from build123d import *

# Parameters (mm, degrees)
CHAMFER_1_SIZE = 1
CHAMFER_2_SIZE = 0.1
CHAMFER_3_SIZE = 0.3


with BuildPart() as part:
    # 스케치1 → 회전1 (revolve)
    with BuildSketch(Plane(origin=(0, 0, 0), x_dir=(0, 0, -1), z_dir=(1, 0, 0))):
        with BuildLine():
            Line((4.2, 0), (4.2, 1))
            Line((4.2, 1), (4.2, 7))
            Line((4.2, 7), (4.7, 7.500000078))
            Line((4.7, 7.500000078), (4.7, 8.000000078))
            Line((4.7, 8.000000078), (4.2, 8.5))
            Line((4.2, 8.5), (4.2, 10))
            Line((4.2, 10), (4.7, 10.500000078))
            Line((4.7, 10.500000078), (4.7, 11.000000078))
            Line((4.7, 11.000000078), (4.2, 11.5))
            Line((4.2, 11.5), (4.2, 13))
            Line((4.2, 13), (4.7, 13.500000078))
            Line((4.7, 13.500000078), (4.7, 14.000000078))
            Line((4.7, 14.000000078), (4.2, 14.5))
            Line((4.2, 14.5), (4.2, 28))
            Line((4.2, 28), (3.533728258, 29.430530536))
            Line((3.533728258, 29.430530536), (2.802745502, 31))
            Line((2.802745502, 31), (2.399244734, 31.778552392))
            ThreePointArc((2.399244734, 31.778552392), (2.719290067, 32.253174869), (2.946609162, 32.778552392))
            Line((2.946609162, 32.778552392), (3.229990685, 33.260397004))
            Line((3.229990685, 33.260397004), (3.229990685, 33.62037773))
            Line((3.229990685, 33.62037773), (3.02, 33.830368416))
            Line((3.02, 33.830368416), (3.02, 34.830368416))
            Line((3.02, 34.830368416), (3.189631584, 35))
            Line((3.189631584, 35), (6, 35))
            Line((6, 35), (6, 25))
            Line((6, 25), (11.05, 10))
            Line((11.05, 10), (11.05, 8))
            Line((11.05, 8), (10.05, 8))
            Line((10.05, 8), (9.5, 7))
            Line((9.5, 7), (9.5, 5))
            Line((9.5, 5), (10.075, 5))
            Line((10.075, 5), (10.075, 1))
            Line((10.075, 1), (9.5, -0.374573668))
            Line((9.5, -0.374573668), (9.5, -2))
            Line((9.5, -2), (4.2, -2))
            Line((4.2, -2), (4.2, 0))
        make_face()
    revolve(axis=Axis((0, 0, 0), (0, 1, 0)))

    # 모따기1
    chamfer_1_edges = [part.edges().sort_by_distance(p)[0] for p in [
        (0, 35, 6),
        (0, -2, 4.2),
    ]]
    chamfer(chamfer_1_edges, length=CHAMFER_1_SIZE)

    # 모따기2
    # the kernel refuses this chamfer: 0.191354542, 0.1 mm, written as the material it takes off along each edge
    with BuildSketch(Plane(origin=(0, 31.778552392, 0), x_dir=(0, 0, -1), z_dir=(1, 0, 0))) as chamfer_2_piece_1:
        with BuildLine():
            Line((2.52619809, 0.166311611), (2.399244734 + CHAMFER_2_SIZE * 0.460143640426, -CHAMFER_2_SIZE * 0.887844485355))
            Line((2.399244734 + CHAMFER_2_SIZE * 0.460143640426, -CHAMFER_2_SIZE * 0.887844485355), (2.399244734, 0))
            ThreePointArc((2.399244734, 0), (2.466310937, 0.08495162), (2.52619809, 0.166311611))
        make_face()
    revolve(axis=Axis((0, 31.778552392, 0), (0, 1, 0)), mode=Mode.SUBTRACT)

    # 모따기3
    chamfer_3_edges = [part.edges().sort_by_distance(p)[0] for p in [
        (0, 8, 11.05),
    ]]
    chamfer(chamfer_3_edges, length=CHAMFER_3_SIZE)


solid = part.part
For this review, take the finished solid that the model builds, in its own axes (mm). A direction names the side the tool comes from. Coordinates: 2 decimals unless noted, no trailing zeros. Loops run counter-clockwise (first coordinate to the right, second up) from the corner with the lowest first, then second, coordinate; pieces in that order, holes last. Notation, with made-up numbers: (-24, 24) - (-10, 24) arc R33 ccw to (-10, 62) - close; hole circle Ø5 at (12, 62). An arc over 180 degrees is marked (long way). Return JSON: item names as keys, results as strings.
Item 1: Mouldability with a two-part tool opening along Z and no side actions: class faces 4 (the cylindrical face through (1.237, 33.443, -2.984)), 5 (the cylindrical face through (-1.262, 9.26, -4.006)), 6 (the cylindrical face through (0, 29, 6)), 7 (the flat face through (1, 35, 3.3)) as pulls with the +Z half, pulls with the -Z half, needs draft (parallel to the pull), parting line crosses it, or undercut.
Determined:
{"face 4": "undercut", "face 5": "undercut", "face 6": "parting line crosses it", "face 7": "needs draft"}
Item 2: Take a section at B-B (y = 16). Give the boundary of the cut face in (x, z), then the cut area to 3 significant figures.
Determined:
{"outline": "circle Ø18.06 at (0, 0); hole circle Ø8.4 at (0, 0)", "area": "201 mm2"}
Item 3: For line 1 (Z direction, x = 0, y = 9); line 2 (X direction, y = 7.6, z = 0); line 3 (Z direction, x = -2.75, y = 1), list the stretches that pass through material, from the lowest coordinate up.
Determined:
{"line 1": "z = -11.05 to -4.2, 4.2 to 11.05", "line 2": "x = -9.83 to -4.7, 4.7 to 9.83", "line 3": "z = -9.69 to -3.17, 3.17 to 9.69"}
Item 4: Insertion check: pin 1 (10 mm diameter, centred on y = 23, z = 5.5, fed in from +X); pin 2 (9.5 mm diameter, centred on x = 0, z = 0, fed in from -Y); pin 3 (7 mm diameter, centred on x = 0, z = 0, fed in from -Y). Each pin has a flat end and moves straight along its axis. Give the tip position at first contact, or say it passes through.
Determined:
{"pin 1": "stops at x = 7.63", "pin 2": "stops at y = -1.55", "pin 3": "stops at y = 29.5"}
Item 5: For faces 1 (the flat face through (9, 5, 4)), 2 (the cylindrical face through (8.43, -1.2, -4.38)), 3 (the flat face through (4, -2, -4)), list the 3-axis set-ups (+Z, -Z, +X, -X, +Y, -Y) from which the entire face can be reached by the end or side of a thin tool; tool diameter is ignored.
Determined:
{"face 1": "none", "face 2": "-Y", "face 3": "+Z, -Z, +X, -X, -Y"}
Item 6: Take a section at A-A (y = 26). Give the boundary of the cut face in (x, z), then the cut area to 3 significant figures.
Determined:
{"outline": "circle Ø12 at (0, 0); hole circle Ø8.4 at (0, 0)", "area": "57.7 mm2"}
